Design review of the part shown in the three views and the two pictorial views. Dimensions are in mm from the part's minimum x, y and z. Coordinates: 2 decimals unless noted, no trailing zeros. Write each loop counter-clockwise with the first axis right and the second up, starting at its lowest first coordinate (ties: lowest second). Pieces come first, ordered by that corner, then holes. Notation, with made-up numbers: M -35.75,4.25 L -30.75,4.25 A8 ccw -30.75,11.25 Z; hole C -31,38.5 d1. An arc over 180 degrees is marked long. Answer as a JSON object with one key per item and string values.
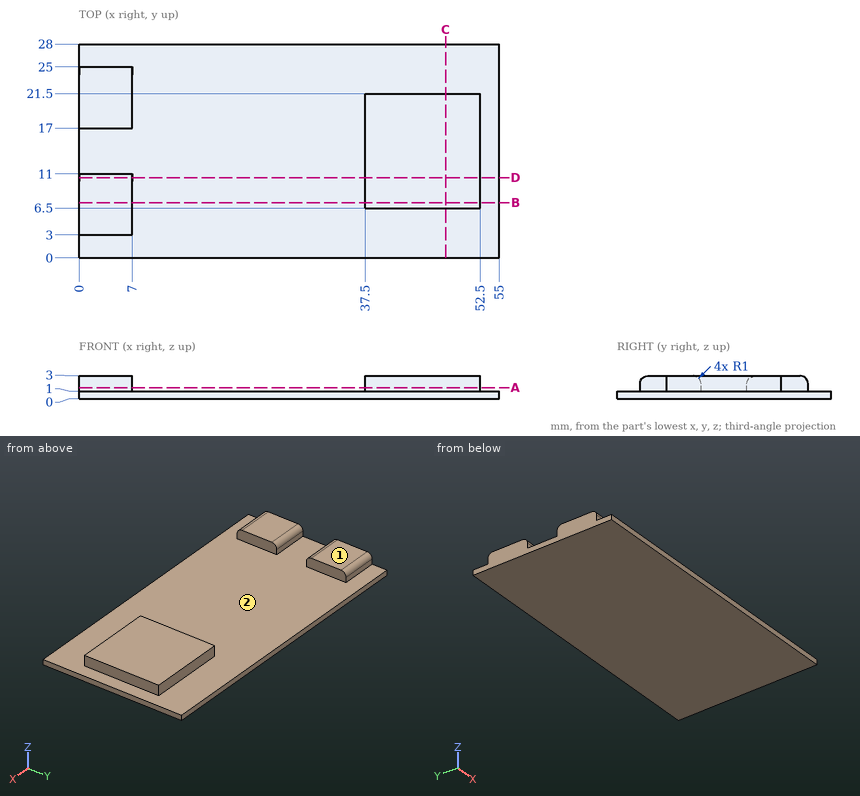
(1) Add section C-C on x = 48. Give the boundary of the cut face in (y, z).
Results list:
{"outline": "M 0,0 L 28,0 L 28,1 L 21.5,1 L 21.5,3 L 6.5,3 L 6.5,1 L 0,1 Z"}
(2) Add section A-A on z = 1.45. Give the boundary of the cut face in (x, y).
Results list:
{"outline": "M 0,3 L 7,3 L 7,11 L 0,11 Z; M 0,17 L 7,17 L 7,25 L 0,25 Z; M 37.5,6.5 L 52.5,6.5 L 52.5,21.5 L 37.5,21.5 Z"}
(3) Wall thickness on line 1 along X through (y, z) = (10.75, 1.1); line 2 along Y through (x, z) = (40.5, 1.5); line 3 along X through (y, z) = (14.5, 1.6): over which ranges is each line inside the solid? List them lowest first. Write a range as from..to.
Results list:
{"line 1": "0..7, 37.5..52.5", "line 2": "6.5..21.5", "line 3": "37.5..52.5"}
(4) Draft analysis for pull direction X (two halves, no side actions). For the marked faces 1 and 2, state which applies: released by +X, released by -X, zero draft, split by the parting line, or undercut.
Results list:
{"face 1": "zero draft", "face 2": "undercut"}
(5) Add section B-B on y = 7.25. Give the boundary of the cut face in (x, z), and give its area (3 significant figures).
Results list:
{"outline": "M 0,0 L 55,0 L 55,1 L 52.5,1 L 52.5,3 L 37.5,3 L 37.5,1 L 7,1 L 7,3 L 0,3 Z", "area": "99.0 mm²"}
(6) For pin 1 Ø1 at (x, y) = (48, 24.5) entering from +Z; pin 2 Ø1.6 at (y, z) = (12, 2) entering from -X; pin 3 Ø1 at (x, z) = (45, 2) entering from -Y, all flat-tipped, find the tip position at first contact; note any pin that passes through.
Results list:
{"pin 1": "z = 1", "pin 2": "x = 37.5", "pin 3": "y = 6.5"}
(7) Add section D-D on y = 10.5. Give the boundary of the cut face in (x, z).
Results list:
{"outline": "M 0,0 L 55,0 L 55,1 L 52.5,1 L 52.5,3 L 37.5,3 L 37.5,1 L 7,1 L 7,2.87 L 0,2.87 Z"}
